```python
from build123d import *

# Parameters (mm, degrees)
SKETCH1_R           = 3.96875
BOSS_EXTRUDE1_DEPTH = 12.7
SKETCH2_R           = 2.38125
CUT_EXTRUDE1_DEPTH  = 7.35


with BuildPart() as part:
    # Sketch1 → Boss-Extrude1 (new body)
    with BuildSketch(Plane(origin=(0, 0, 0), x_dir=(0, 0, -1), z_dir=(1, 0, 0))):
        with BuildLine():
            Line((-26.587134527, 4.994963407), (-26.587134527, -2.625036593))
            Line((-26.587134527, -2.625036593), (-32.937134527, -2.625036593))
            Line((-32.937134527, -2.625036593), (-32.937134527, 22.774963407))
            Line((-32.937134527, 22.774963407), (-26.587134527, 22.774963407))
            Line((-26.587134527, 22.774963407), (-26.587134527, 15.154963407))
            Line((-26.587134527, 15.154963407), (-18.967134527, 15.154963407))
            ThreePointArc((-18.967134527, 15.154963407), (-13.887134527, 10.074963407), (-18.967134527, 4.994963407))
            Line((-18.967134527, 4.994963407), (-26.587134527, 4.994963407))
        make_face()
        with Locations((-18.967134527, 10.074963407)):
            Circle(SKETCH1_R, mode=Mode.SUBTRACT)
    extrude(amount=BOSS_EXTRUDE1_DEPTH)

    # Sketch2 → Cut-Extrude1 (cut, through all)
    with BuildSketch(Plane(origin=(0, 0, 26.587134527), x_dir=(-1, 0, 0), z_dir=(0, 0, -1))):
        with Locations((-6.35, 18.964963407)):
            Circle(SKETCH2_R)
        with Locations((-6.35, 1.184963407)):
            Circle(SKETCH2_R)
    extrude(amount=-CUT_EXTRUDE1_DEPTH, mode=Mode.SUBTRACT)


solid = part.part
```
The listing builds one solid part. Answer for the finished solid, in the listing's coordinates (mm). A direction names the side the tool comes from. Round coordinates to 2 decimals unless told otherwise and drop trailing zeros. Order: outer loops, then holes, each group sorted by start corner. A loop starts at its lowest first (then second) coordinate and runs counter-clockwise, first axis right, second up. Notation, with made-up numbers: (86, 84.5) -> (126, 84.5) arc R5 ccw to (126, 91.5) -> close; hole circle Ø10 at (87.5, 29.5). An arc over 180 degrees is marked (long way). Answer as CSV lines item,"result". Start each with the question number.
(1) Flat-ended cylindrical pins translate along their axes: pin 1 Ø4 at (x, y) = (6.5, 0) entering from -Z; pin 2 Ø6 at (x, z) = (4, 17) entering from -Y; pin 3 Ø10.5 at (y, z) = (10.07, 18.97) entering from -X; pin 4 Ø1.5 at (x, z) = (5, 17.5) entering from +Y. Find the tip coordinate at first contact, or state that the pin passes through.
(2) The part is cut by section C-C (y = -0.5). Determine the outline of the cut face in (x, z), then the cut area to 3 significant figures.
(3) The part is cut by section D-D (x = 5). Determine the outline of the cut face in (y, z).
(4) Find the intervals of material crossed by probe 1 along Y at (x, z) = (6.35, 28.5); probe 2 along Z at (x, y) = (5.25, 10.25); probe 3 along Y at (x, z) = (5, 18.75), in increasing order. Write a range as from..to.
(5) For a pull along Y with two mould halves and no side action, classify faces 1 (the face through (6, 4.995, 23)), 2 (the face through (6.87, 16.64, 29.72)), 3 (the face through (6, 22, 26.587)) as +Y half, -Y half, draft (parallel to the pull), parting line (faces both ways), or undercut.
(6) The part is cut by section B-B (z = 20). Determine the outline of the cut face in (x, y).
(7) The part is cut by section A-A (x = 7.75). Determine the outline of the cut face in (y, z).
(8) A tool of negligible diameter and unlimited length cuts with its end or side. For faces 4 (the face through (6, 22.775, 30)), 5 (the face through (6, 15.155, 23)), 6 (the face through (6, 4, 26.587)), from which of +Z, -Z, +X, -X, +Y, -Y can it reach the whole face along a straight path? Write none if from no direction.
Evaluation:
1,pin 1,"z = 26.59"
1,pin 2,"y = 4.99"
1,pin 3,"x = 0"
1,pin 4,"y = 15.1"
2,outline,"(0, 26.59) -> (4.67, 26.59) -> (4.67, 32.94) -> (0, 32.94) -> close; (8.03, 26.59) -> (12.7, 26.59) -> (12.7, 32.94) -> (8.03, 32.94) -> close"
2,area,"59.3 mm²"
3,outline,"(-2.63, 26.59) -> (-0.78, 26.59) -> (-0.78, 32.94) -> (-2.63, 32.94) -> close; (3.15, 26.59) -> (4.99, 26.59) -> (4.99, 18.97) arc R5.08 ccw to (15.15, 18.97) -> (15.15, 26.59) -> (17, 26.59) -> (17, 32.94) -> (3.15, 32.94) -> close; (20.93, 26.59) -> (22.77, 26.59) -> (22.77, 32.94) -> (20.93, 32.94) -> close; hole circle Ø7.94 at (10.07, 18.97)"
4,probe 1,"-2.63..-1.2, 3.57..16.58, 21.35..22.77"
4,probe 2,"13.89..15, 22.93..32.94"
4,probe 3,"5..6.11, 14.04..15.15"
5,face 1,"-Y half"
5,face 2,"undercut"
5,face 3,"draft"
6,outline,"(0, 4.99) -> (12.7, 4.99) -> (12.7, 6.24) -> (0, 6.24) -> close; (0, 13.91) -> (12.7, 13.91) -> (12.7, 15.15) -> (0, 15.15) -> close"
7,outline,"(-2.63, 26.59) -> (-0.74, 26.59) -> (-0.74, 32.94) -> (-2.63, 32.94) -> close; (3.11, 26.59) -> (4.99, 26.59) -> (4.99, 18.97) arc R5.08 ccw to (15.15, 18.97) -> (15.15, 26.59) -> (17.04, 26.59) -> (17.04, 32.94) -> (3.11, 32.94) -> close; (20.89, 26.59) -> (22.77, 26.59) -> (22.77, 32.94) -> (20.89, 32.94) -> close; hole circle Ø7.94 at (10.07, 18.97)"
8,face 4,"+Z, -Z, +X, -X, +Y"
8,face 5,"-Z, +X, -X, +Y"
8,face 6,"-Z, +X, -X, -Y"
